Could you check a few things on this model? Use its own coordinates, in mm. Face numbers are marked on the shaded views. Give positions to 0.01 mm unless a question says otherwise; leave off trailing zeros. Loops run counter-clockwise (first coordinate to the right, second up) from the corner with the lowest first, then second, coordinate; pieces in that order, holes last. Notation, with made-up numbers: (-15, -17.5) - (13, -17.5) arc R25 ccw to (13, 5.5) - close; hole circle Ø9 at (25.5, 71). An arc over 180 degrees is marked (long way). One line per item, written item: value. Start each with the question number.
Q1. If we mould it in two halves opening along X, with no side actions, what happens to the marked faces 1, 2 and 3? For each: released by +X, released by -X, zero draft, split by the parting line, or undercut.
Q2. If I drill on line 1 (Z direction, x = 43, y = 29); line 2 (Z direction, x = 72, y = 80); line 3 (Y direction, x = 26.5, z = 934.5), over which ranges is the centre line in solid material (lowest first)? Write a range as from..to.
Q3. I'm going to push flat-ended pins straight in: P1, Ø8, axis at x = 41, z = 623.5, coming from the -Y side; P2, Ø6, axis at x = 78, y = 48, coming from the -Z side; P3, Ø13.5, axis at x = 35, y = 16.5, coming from the +Z side. Where does each tip first touch, or does it pass through?
Q4. I want a section at B-B (x = 36). Please give me the cut outline in (y, z).
Q5. I want a section at A-A (y = 54). Please give me the cut outline in (x, z), then the cut area to 4 significant figures.
```python
from build123d import *

# Parameters (mm, degrees)
SKETCH1_W           = 90
SKETCH1_H           = 90
BOSS_EXTRUDE1_DEPTH = 1000
SKETCH3_W           = 90
SKETCH3_H           = 90
CUT_EXTRUDE1_DEPTH  = 45
SKETCH4_W           = 90
SKETCH4_H           = 90
CUT_EXTRUDE2_DEPTH  = 45


with BuildPart() as part:
    # Sketch1 → Boss-Extrude1 (new body)
    with BuildSketch(Plane.XY):
        with Locations((45, 45)):
            Rectangle(SKETCH1_W, SKETCH1_H)
    extrude(amount=BOSS_EXTRUDE1_DEPTH)

    # Sketch3 → Cut-Extrude1 (cut)
    with BuildSketch(Plane.XZ):
        with Locations((45, 955)):
            Rectangle(SKETCH3_W, SKETCH3_H)
    extrude(amount=-CUT_EXTRUDE1_DEPTH, mode=Mode.SUBTRACT)

    # Sketch4 → Cut-Extrude2 (cut)
    with BuildSketch(Plane(origin=(90, 0, 0), x_dir=(0, 0, -1), z_dir=(1, 0, 0))):
        with Locations((-45, 45)):
            Rectangle(SKETCH4_W, SKETCH4_H)
    extrude(amount=-CUT_EXTRUDE2_DEPTH, mode=Mode.SUBTRACT)


solid = part.part
```
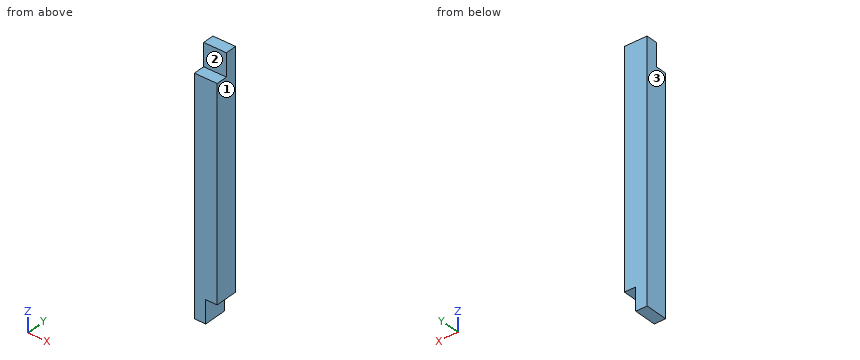
Worked answers:
1. face 1: released by +X
1. face 2: zero draft
1. face 3: released by -X
2. line 1: z = 0..910
2. line 2: z = 90..1000
2. line 3: y = 45..90
3. P1: stops at y = 0
3. P2: stops at z = 90
3. P3: stops at z = 910
4. outline: (0, 0) - (90, 0) - (90, 1000) - (45, 1000) - (45, 910) - (0, 910) - close
5. outline: (0, 0) - (45, 0) - (45, 90) - (90, 90) - (90, 1000) - (0, 1000) - close
5. area: 85,950 mm²
